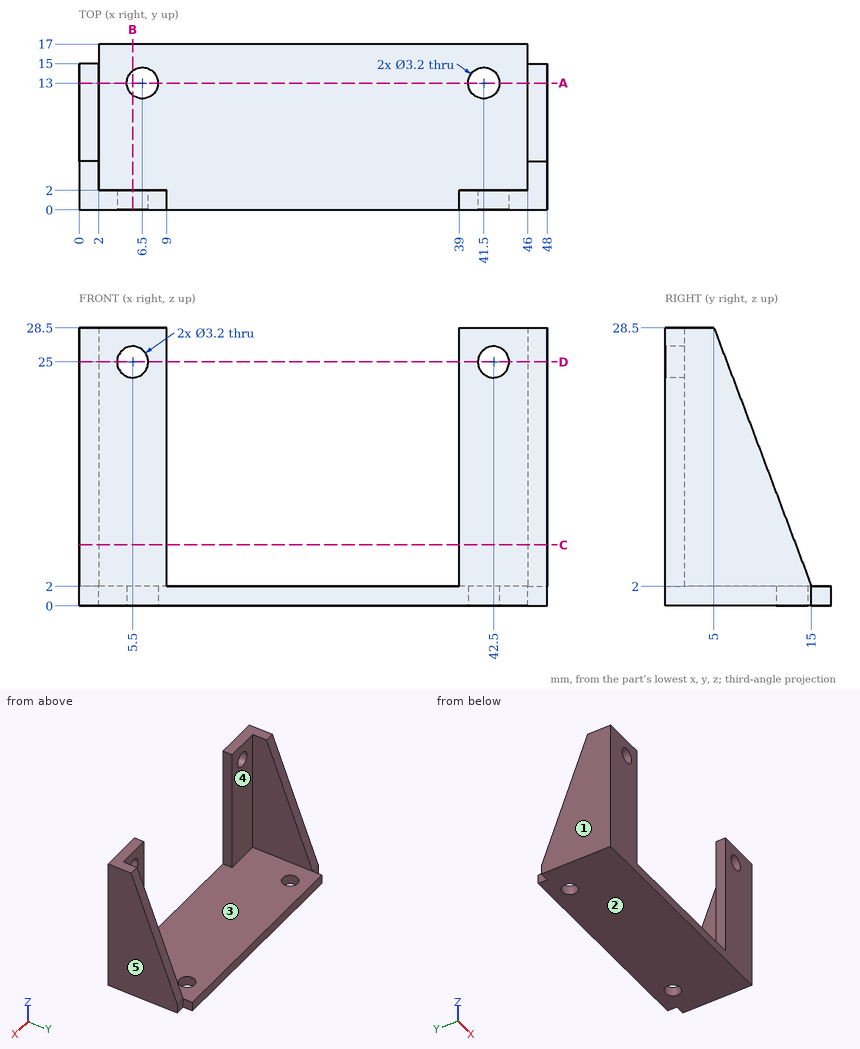
Study the drawing (mm; zero at the part's minimum x, y, z) and answer. A direction names the side the tool comes from. Give positions to 0.01 mm unless a question says otherwise; leave off trailing zeros. Write each loop counter-clockwise with the first axis right and the second up, starting at its lowest first coordinate (ties: lowest second). Pieces come first, ordered by that corner, then holes. Notation, with made-up numbers: (71.5, 86) - (119.5, 86) arc R21 cw to (119.5, 118) - close; hole circle Ø11 at (25, 29.5). An arc over 180 degrees is marked (long way). One line per question, with ' | ' between items. Start each with the question number.
1. For the marked faces 4 and 5, determine the directions among +Z, -Z, +X, -X, +Y, -Y from which every point of the face is accessible in a straight line to the end or side of a thin tool.
2. Section B-B, the plane x = 5.5 is taken. Determine the outline of the cut face in (y, z).
3. Straight lines are drawn through the part: line 1 (X direction, y = 13, z = 0.45); line 2 (X direction, y = 12.5, z = 2.25); line 3 (Z direction, x = 5.5, y = 0.8). For each, find the intervals that lie inside material, in ascending order.
4. Given P1, Ø3, axis at x = 42.5, z = 25, coming from the -Y side; P2, Ø1, axis at x = 47, z = 1, coming from the +Y side; P3, Ø5.5, axis at x = 6, z = 19, coming from the +Y side; P4, Ø1, axis at y = 16.5, z = 0.5, coming from the +X side, each flat-ended and moving along its own axis, determine where each tip first touches the part or whether it passes through.
5. Section A-A, the plane y = 13 is taken. Determine the outline of the cut face in (x, z).
6. Section C-C, the plane z = 6.25 is taken. Determine the outline of the cut face in (x, y), then the cut area to 3 significant figures.
7. Determine the mould class of the marked faces 1, 2 and 3 for opening direction X: +X half, -X half, draft (parallel to the pull), parting line (faces both ways), or undercut.
8. Section D-D, the plane z = 25 is taken. Determine the outline of the cut face in (x, y), then the cut area to 3 significant figures.
Result:
1) face 4: +Z, +Y | face 5: +Z, -Z, +X, +Y, -Y
2) outline: (0, 0) - (11.75, 0) - (11.75, 2) - (2, 2) - (2, 23.4) - (0, 23.4) - close; (0, 26.6) - (2, 26.6) - (2, 28.5) - (0, 28.5) - close; (14.25, 0) - (17, 0) - (17, 2) - (14.25, 2) - close
3) line 1: x = 0 to 4.9, 8.1 to 39.9, 43.1 to 48 | line 2: x = 0 to 2, 46 to 48 | line 3: z = 0 to 23.4, 26.6 to 28.5
4) P1: passes through | P2: stops at y = 15 | P3: stops at y = 2 | P4: stops at x = 46
5) outline: (0, 0) - (4.9, 0) - (4.9, 2) - (2, 2) - (2, 7.3) - (0, 7.3) - close; (8.1, 0) - (39.9, 0) - (39.9, 2) - (8.1, 2) - close; (43.1, 0) - (48, 0) - (48, 7.3) - (46, 7.3) - (46, 2) - (43.1, 2) - close
6) outline: (0, 0) - (9, 0) - (9, 2) - (2, 2) - (2, 13.4) - (0, 13.4) - close; (39, 0) - (48, 0) - (48, 13.4) - (46, 13.4) - (46, 2) - (39, 2) - close | area: 81.6 mm2
7) face 1: -X half | face 2: draft | face 3: undercut
8) outline: (0, 0) - (3.9, 0) - (3.9, 2) - (2, 2) - (2, 6.32) - (0, 6.32) - close; (7.1, 0) - (9, 0) - (9, 2) - (7.1, 2) - close; (39, 0) - (40.9, 0) - (40.9, 2) - (39, 2) - close; (44.1, 0) - (48, 0) - (48, 6.32) - (46, 6.32) - (46, 2) - (44.1, 2) - close | area: 40.5 mm2
